Could you check a few things on this model? Use its own coordinates, in mm. Face numbers are marked on the shaded views. Give positions to 0.01 mm unless a question says otherwise; leave off trailing zeros. Loops run counter-clockwise (first coordinate to the right, second up) from the corner with the lowest first, then second, coordinate; pieces in that order, holes last. Notation, with made-up numbers: (35, -18) - (41, -18) arc R29 cw to (41, 3) - close; hole circle Ø2 at (13, 9.5). An arc over 180 degrees is marked (long way). One line per item, written item: value. Start each with the question number.
Q1. If we mould it in two halves opening along Y, with no side actions, what happens to the marked faces 1, 2 and 3? For each: released by +Y, released by -Y, zero draft, split by the parting line, or undercut.
Q2. If I drill on line 1 (Z direction, x = 0, y = -14); line 2 (Y direction, x = -11, z = 42); line 3 (Z direction, x = 1.5, y = -13), over which ranges is the centre line in solid material (lowest first)? Write a range as from..to.
Q3. I want a section at D-D (x = -19.5). Please give me the cut outline in (y, z).
Q4. I'm going to push flat-ended pins straight in: P1, Ø15, axis at x = -2.5, z = 5.5, coming from the -Y side; P2, Ø10, axis at y = -12, z = -43.5, coming from the -X side. Where does each tip first touch, or does it pass through?
Q5. I want a section at B-B (y = -19.5). Please give me the cut outline in (x, z).
Q6. I want a section at C-C (y = -36). Please give me the cut outline in (x, z), then the cut area to 3 significant figures.
Q7. I want a section at A-A (z = 0). Please give me the cut outline in (x, y), then the cut area to 3 significant figures.
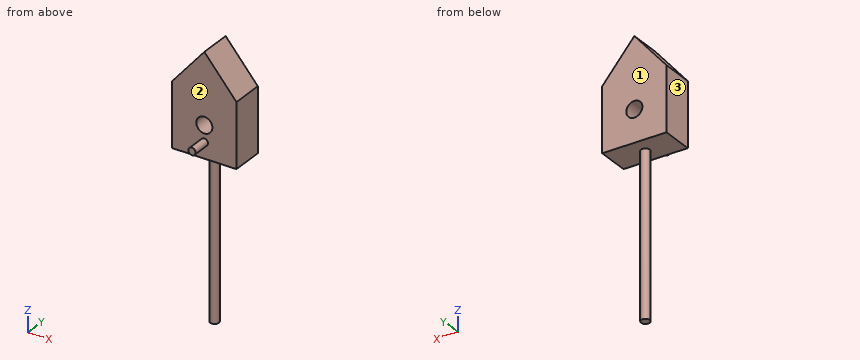
```python
from build123d import *

# Parameters (mm, degrees)
F0_R     = 6.35
F1_DEPTH = 25.4
F2_R     = 2.87548
F3_DEPTH = 14.732
F4_R     = 3.475255
F5_DEPTH = 129.032


with BuildPart() as f1:
    # F0 (on Front) → F1 (new body)
    with BuildSketch(Plane.XZ):
        Polygon((-25.4, -25.4), (25.4, -25.4), (25.4, 25.4), (0, 55.480507), (-25.4, 25.4), align=None)
        Circle(F0_R, mode=Mode.SUBTRACT)
    extrude(amount=F1_DEPTH)

    # F2 (on face) → F3 (join)
    with BuildSketch(Plane.XZ.offset(25.4)):
        with Locations((0, -12.954)):
            Circle(F2_R)
    extrude(amount=F3_DEPTH)

    # F4 (on face) → F5 (join)
    with BuildSketch(Plane(origin=(0, 0, -25.4), x_dir=(1, 0, 0), z_dir=(0, 0, -1))):
        with Locations((0, 13.2588)):
            Circle(F4_R)
    extrude(amount=F5_DEPTH)


solid = f1.part
```
Worked answers:
1. face 1: released by +Y
1. face 2: released by -Y
1. face 3: zero draft
2. line 1: z = -154.43..-6.35, 6.35..55.48
2. line 2: y = -25.4..0
2. line 3: z = -154.43..-6.17, 6.17..53.7
3. outline: (-25.4, -25.4) - (0, -25.4) - (0, 32.39) - (-25.4, 32.39) - close
4. P1: stops at y = -25.4
4. P2: stops at x = -3.48
5. outline: (-25.4, -25.4) - (25.4, -25.4) - (25.4, 25.4) - (0, 55.48) - (-25.4, 25.4) - close; hole circle Ø12.7 at (0, 0)
6. outline: circle Ø5.75 at (0, -12.95)
6. area: 26.0 mm²
7. outline: (-25.4, -25.4) - (-6.35, -25.4) - (-6.35, 0) - (-25.4, 0) - close; (6.35, -25.4) - (25.4, -25.4) - (25.4, 0) - (6.35, 0) - close
7. area: 968 mm²
